The listing builds one solid part. Answer for the finished solid, in the listing's coordinates (mm). Coordinates: 2 decimals unless noted, no trailing zeros. Order: outer loops, then holes, each group sorted by start corner. A loop starts at its lowest first (then second) coordinate and runs counter-clockwise, first axis right, second up. Notation, with made-up numbers: M -5.75,52 L 0.25,52 A21 cw 0.25,86 Z; hole C 63,19.25 d8. An arc over 180 degrees is marked long. One line per item, written item: value. Start each with the question number.
Q1. The part is cut by section C-C on z = 3.1. Give the vertices of the cut face in (x, y), then the cut area to 3 significant figures.
Q2. Straight lines are drawn through the part: line 1 along X through (y, z) = (59, 1.35); line 2 along X through (y, z) = (39.5, 0.95); line 3 along X through (y, z) = (47.5, 1.1). For each, find the intervals that lie inside material, in ascending order. Write a range as [from, to].
Q3. Each of these flat-tipped pins is pushed along its axis until it touches: pin 1 Ø10.5 at (x, y) = (3, 10.5) entering from -Z; pin 2 Ø1.5 at (y, z) = (59.5, 2.5) entering from +X. Where does it stop, or does it pass through?
```python
from build123d import *

# Parameters (mm, degrees)
SKETCH002_R     = 2.6
PAD001_DEPTH    = 2
PAD002_DEPTH    = 2
POCKET003_DEPTH = 2.201
PAD003_DEPTH    = 2.2
POCKET004_DEPTH = 4.001
SKETCH006_R     = 17.1
SKETCH006_R_2   = 14.9
POCKET002_DEPTH = 1
CHAMFER002_SIZE = 0.4
CHAMFER_SIZE    = 1.99
SKETCH004_R     = 2.2
POCKET_DEPTH    = 4.001
SKETCH005_R     = 6.2
POCKET001_DEPTH = 2.001
SKETCH010_R     = 4
POCKET005_DEPTH = 1
CHAMFER001_SIZE = 1.7
POCKET006_DEPTH = 5


with BuildPart() as part:
    # Sketch002 → Pad001 (new body)
    with BuildSketch(Plane.XY):
        Polygon((-116.824546, 67.621888), (-37.5, 205.016032), (37.5, 205.016032), (116.824546, 67.621888), (0, 0.173205), align=None)
        with Locations((-51.370835, 167.991041)):
            Circle(SKETCH002_R, mode=Mode.SUBTRACT)
        with Locations((51.370835, 167.991041)):
            Circle(SKETCH002_R, mode=Mode.SUBTRACT)
    extrude(amount=PAD001_DEPTH)

    # Sketch003 → Pad002 (join)
    with BuildSketch(Plane.XY.offset(2)):
        Polygon((-118.899546, 64.027883), (-114.899546, 70.956086), (-0.173205, 4.718802), (-0.173205, 0.1), (-4.173205, -2.209401), align=None)
    extrude(amount=PAD002_DEPTH)

    # Sketch007 → Pocket003 (cut, through all)
    with BuildSketch(Plane.XY.offset(2.2)):
        Polygon((-116.824546, 67.621888), (0, 0.173205), (-4.173205, -2.209401), (-118.899546, 64.027883), align=None)
    extrude(amount=-POCKET003_DEPTH, mode=Mode.SUBTRACT)

    # Sketch008 → Pad003 (join)
    with BuildSketch(Plane.XY):
        Polygon((-104.909165, 58.259933), (-87.588657, 48.259933), (-88.588657, 46.527883), (-105.909165, 56.527883), align=None)
    extrude(amount=PAD003_DEPTH)

    # Sketch009 → Pocket004 (cut, through all)
    with BuildSketch(Plane.XY):
        Polygon((83.830836, 53.168669), (84.960836, 51.211452), (103.666985, 62.011452), (102.536985, 63.968669), align=None)
    extrude(amount=POCKET004_DEPTH, mode=Mode.SUBTRACT)

    # Sketch006 → Pocket002 (cut)
    with BuildSketch(Plane.XY):
        Circle(SKETCH006_R)
        Circle(SKETCH006_R_2, mode=Mode.SUBTRACT)
    extrude(amount=POCKET002_DEPTH, mode=Mode.SUBTRACT)

    # Chamfer002
    chamfer002_edges = [part.edges().sort_by_distance(p)[0] for p in [
        (-96.248911, 53.259933, 0),
        (-88.088657, 47.393908, 0),
        (-97.248911, 51.527883, 0),
        (-105.409165, 57.393908, 0),
        (94.313911, 56.611452, 0),
        (103.101985, 62.99006, 0),
        (93.183911, 58.568669, 0),
        (84.395836, 52.19006, 0),
        (0, 14.9, 0),
        (0, 17.1, 0),
    ]]
    chamfer(chamfer002_edges, length=CHAMFER002_SIZE)

    # Chamfer
    chamfer_edges = [part.edges().sort_by_distance(p)[0] for p in [
        (-57.536375, 37.837444, 4),
    ]]
    chamfer(chamfer_edges, length=CHAMFER_SIZE)

    # Sketch004 → Pocket (cut, through all)
    with BuildSketch(Plane.XY):
        Circle(SKETCH004_R)
    extrude(amount=POCKET_DEPTH, mode=Mode.SUBTRACT)

    # Sketch005 → Pocket001 (cut, through all)
    with BuildSketch(Plane.XY.offset(2)):
        Circle(SKETCH005_R)
    extrude(amount=POCKET001_DEPTH, mode=Mode.SUBTRACT)

    # Sketch010 → Pocket005 (cut)
    with BuildSketch(Plane.XY.offset(2)):
        with Locations((-51.370835, 167.991041)):
            Circle(SKETCH010_R)
        with Locations((51.370835, 167.991041)):
            Circle(SKETCH010_R)
    extrude(amount=-POCKET005_DEPTH, mode=Mode.SUBTRACT)

    # Chamfer001
    chamfer001_edges = [part.edges().sort_by_distance(p)[0] for p in [
        (-5.849077, 2.056283, 4),
        (-62.500992, 31.466162, 4),
        (-117.397046, 66.630289, 4),
    ]]
    chamfer(chamfer001_edges, length=CHAMFER001_SIZE)

    # Sketch011 → Pocket006 (cut)
    with BuildSketch(Plane.XY):
        with BuildLine():
            Line((-112.899546, 74.420187), (-37.5, 205.016032))
            Line((-37.5, 205.016032), (37.5, 205.016032))
            Line((37.5, 205.016032), (112.899546, 74.420187))
            Line((112.899546, 74.420187), (11.968954, 16.147883))
            ThreePointArc((11.968954, 16.147883), (0, 20.1), (-11.968954, 16.147883))
            Line((-11.968954, 16.147883), (-112.899546, 74.420187))
        make_face()
    extrude(amount=POCKET006_DEPTH, mode=Mode.SUBTRACT)


solid = part.part
```
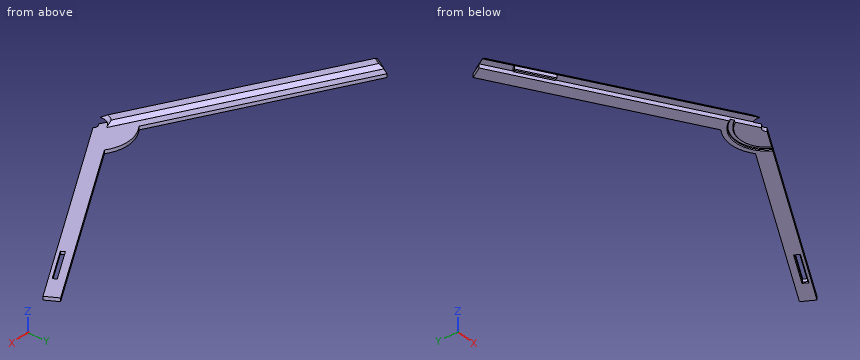
Output:
1. outline: M -117.81,64.32 L -6.99,0.34 A7 cw -4.06,5.7 L -114.75,69.61 Z
1. area: 779 mm^2
2. line 1: x = [-101.89, -86.19], [86.19, 93.93], [98.45, 101.89]
2. line 2: x = [-68.12, -52.42], [52.42, 68.12]
2. line 3: x = [-90.27, -88.03], [-81.97, -66.27], [66.27, 81.97]
3. pin 1: stops at z = 0
3. pin 2: stops at x = 103.73
